```python
from build123d import *

# Parameters (mm, degrees)
SKETCH1_R           = 10.5
SKETCH1_R_2         = 8.0375
BOSS_EXTRUDE1_DEPTH = 5
BOSS_EXTRUDE2_START = -5
SKETCH1_3_R         = 8.0375
SKETCH1_3_R_2       = 6.75
BOSS_EXTRUDE2_DEPTH = 2
CHAMFER1_SIZE       = 1


with BuildPart() as part:
    # Sketch1 → Boss-Extrude1 (new body, symmetric)
    with BuildSketch(Plane.XY):
        Circle(SKETCH1_R)
        Circle(SKETCH1_R_2, mode=Mode.SUBTRACT)
    extrude(amount=BOSS_EXTRUDE1_DEPTH, both=True)

    # Sketch1<3> → Boss-Extrude2 (add)
    with BuildSketch(Plane.XY.offset(BOSS_EXTRUDE2_START)):
        Circle(SKETCH1_3_R)
        Circle(SKETCH1_3_R_2, mode=Mode.SUBTRACT)
    extrude(amount=BOSS_EXTRUDE2_DEPTH)

    # Chamfer1
    chamfer1_edges = [part.edges().sort_by_distance(p)[0] for p in [
        (-8.0375, 0, 5),
    ]]
    chamfer(chamfer1_edges, length=CHAMFER1_SIZE)


solid = part.part
```
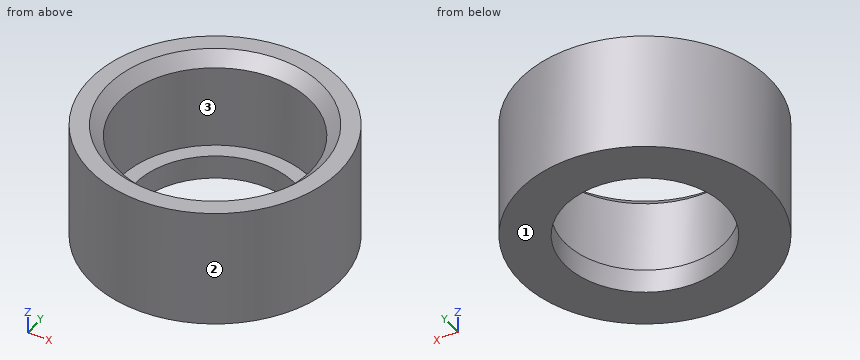
CAD build for the part. Positions are in the model's coordinates, mm. Face numbers are marked on the shaded views. Round coordinates to 2 decimals unless told otherwise and drop trailing zeros. Order: outer loops, then holes, each group sorted by start corner. A loop starts at its lowest first (then second) coordinate and runs counter-clockwise, first axis right, second up.
Item 1: Pin check, flat tips, straight feed: pin 1 (12 mm diameter, centred on x = 0, y = 0, fed in from +Z); pin 2 (4 mm diameter, centred on x = 6.5, z = -3.5, fed in from +Y); pin 3 (1 mm diameter, centred on y = -6, z = 3.5, fed in from +X); pin 4 (2 mm diameter, centred on x = -1, y = 6, fed in from +Z). Stop position of each tip, or through.
Item 2: Saw through at C-C on z = -2.5. Write the cut outline in (x, y) (1 decimal), then the cut area to 3 significant figures.
Item 3: Mould opens along X. For the marked faces 1, 2 and 3 say: pulls with the +X half, pulls with the -X half, needs draft (parallel to the pull), parting line crosses it, or undercut.
Item 4: Probe line 1 along Y through (x, z) = (0, 1); line 2 along X through (y, z) = (-5.5, 3.25); line 3 along X through (y, z) = (-2.75, -4). List the from-to ranges inside material, lowest first.
Item 5: Saw through at A-A on x = 0. Write the cut outline in (y, z), then the cut area to 3 significant figures.
Reported:
1. pin 1: passes through
1. pin 2: stops at y = 9.49
1. pin 3: stops at x = 8.94
1. pin 4: stops at z = -3
2. outline: circle Ø21 at (0, 0); hole circle Ø16.1 at (0, 0)
2. area: 143 mm2
3. face 1: needs draft
3. face 2: parting line crosses it
3. face 3: undercut
4. line 1: y = -10.5 to -8.04, 8.04 to 10.5
4. line 2: x = -8.94 to -5.86, 5.86 to 8.94
4. line 3: x = -10.13 to -6.16, 6.16 to 10.13
5. outline: (-10.5, -5) - (-6.75, -5) - (-6.75, -3) - (-8.04, -3) - (-8.04, 4) - (-9.04, 5) - (-10.5, 5) - close; (6.75, -5) - (10.5, -5) - (10.5, 5) - (9.04, 5) - (8.04, 4) - (8.04, -3) - (6.75, -3) - close
5. area: 53.4 mm2
